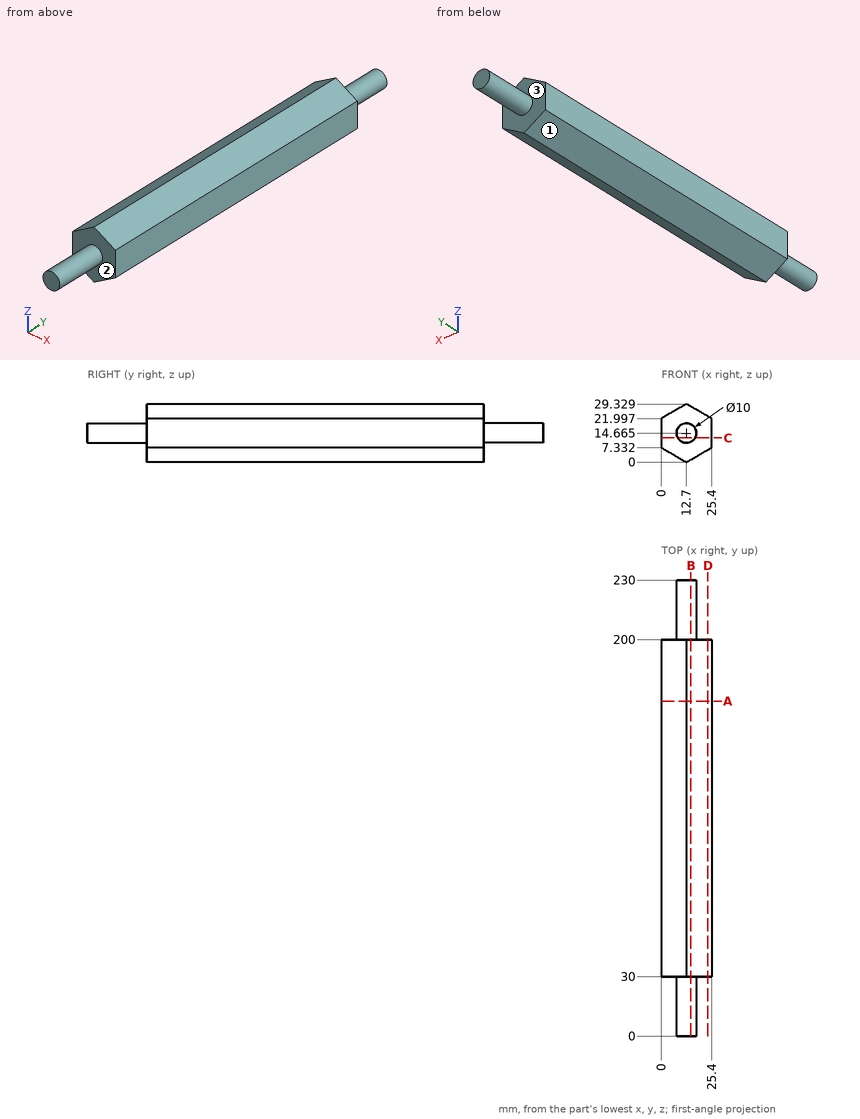
Answer from the drawing. Dimensions are ordinates in mm from the lowest x, y and z of the part. A direction names the side the tool comes from. Round coordinates to 2 decimals unless told otherwise and drop trailing zeros. Order: outer loops, then holes, each group sorted by start corner. A loop starts at its lowest first (then second) coordinate and runs counter-clockwise, first axis right, second up. Notation, with made-up numbers: (24, -21.75) - (44, -21.75) arc R18 cw to (44, -3.75) - close; hole circle Ø1 at (67, -1). An arc over 180 degrees is marked (long way). Put each result on its own line as item: value. Start each with the question number.
(1) Given P1, Ø5, axis at x = 12.5, y = 65, coming from the +Z side; P2, Ø12, axis at x = 4.5, z = 23, coming from the -Y side; P3, Ø1.5, axis at y = 202.5, z = 18.5, coming from the +X side (1 decimal); P4, Ø1, axis at x = 8.5, y = 30, coming from the +Z side, each flat-ended and moving along its own axis, determine where each tip first touches the part or whether it passes through.
(2) For the marked faces 1, 2 and 3, determine the directions among +Z, -Z, +X, -X, +Y, -Y from which every point of the face is accessible in a straight line to the end or side of a thin tool.
(3) Straight lines are drawn through the part: probe 1 along Y at (x, z) = (13.25, 5.75); probe 2 along Z at (x, y) = (12.75, 23) (1 decimal); probe 3 along X at (y, z) = (26.5, 14) (1 decimal). For each, find the intervals that lie inside material, in ascending order. Write a range as from..to.
(4) Find section A-A (y = 169). Give the vertices of the cut face in (x, z).
(5) Find section D-D (x = 23.5). Give the vertices of the cut face in (y, z) (1 decimal).
(6) Find section C-C (z = 12.25). Give the vertices of the cut face in (x, y), plus the area to 3 significant figures.
(7) Find section B-B (x = 15). Give the vertices of the cut face in (y, z) (1 decimal), plus the area to 3 significant figures.
Reply:
1. P1: z = 29.33
1. P2: y = 30
1. P3: x = 16.6
1. P4: z = 27.19
2. face 1: -Z, -X, +Y, -Y
2. face 2: -Y
2. face 3: +Y
3. probe 1: 30..200
3. probe 2: 9.7..19.7
3. probe 3: 7.7..17.7
4. outline: (0, 7.33) - (12.7, 0) - (25.4, 7.33) - (25.4, 22) - (12.7, 29.33) - (0, 22) - close
5. outline: (30, 6.2) - (200, 6.2) - (200, 23.1) - (30, 23.1) - close
6. outline: (0, 30) - (8.32, 30) - (8.32, 0) - (17.08, 0) - (17.08, 30) - (25.4, 30) - (25.4, 200) - (17.08, 200) - (17.08, 230) - (8.32, 230) - (8.32, 200) - (0, 200) - close
6. area: 4,840 mm^2
7. outline: (0, 10.2) - (30, 10.2) - (30, 1.3) - (200, 1.3) - (200, 10.2) - (230, 10.2) - (230, 19.1) - (200, 19.1) - (200, 28) - (30, 28) - (30, 19.1) - (0, 19.1) - close
7. area: 5,070 mm^2
